Check sheet for the modelled part. Datum: model origin and axes. Units: mm. Face numbers are marked on the shaded views. A direction names the side the tool comes from. Round coordinates to 2 decimals unless told otherwise and drop trailing zeros. Loops run counter-clockwise (first coordinate to the right, second up) from the corner with the lowest first, then second, coordinate; pieces in that order, holes last. Notation, with made-up numbers: (73.5, -18.75) -> (85.5, -18.75) arc R22 ccw to (85.5, -3.75) -> close; hole circle Ø11 at (-39, 24). An arc over 180 degrees is marked (long way). Return JSON: item names as keys, results as strings.
from build123d import *

# Parameters (mm, degrees)
SKETCH2_W           = 61
SKETCH2_H           = 42.5
SKETCH2_R           = 11.5
SKETCH2_R_2         = 1.75
BOSS_EXTRUDE2_DEPTH = 5
BOSS_EXTRUDE3_DEPTH = 3
LPATTERN1_COUNT     = 2
LPATTERN1_PITCH     = 45.5


with BuildPart() as part:
    # Sketch2 → Boss-Extrude2 (new body)
    with BuildSketch(Plane(origin=(0, 0, 0), x_dir=(0, 0, -1), z_dir=(1, 0, 0))):
        with Locations((9.5, 0)):
            Rectangle(SKETCH2_W, SKETCH2_H)
        Circle(SKETCH2_R, mode=Mode.SUBTRACT)
        with Locations((-15.5, 15.5)):
            Circle(SKETCH2_R_2, mode=Mode.SUBTRACT)
        with Locations((15.5, -15.5)):
            Circle(SKETCH2_R_2, mode=Mode.SUBTRACT)
        with Locations((15.5, 15.5)):
            Circle(SKETCH2_R_2, mode=Mode.SUBTRACT)
        with Locations((-15.5, -15.5)):
            Circle(SKETCH2_R_2, mode=Mode.SUBTRACT)
        with BuildLine():
            Line((28.5, 12.75), (31.5, 12.75))
            ThreePointArc((31.5, 12.75), (34.25, 10), (31.5, 7.25))
            Line((31.5, 7.25), (28.5, 7.25))
            ThreePointArc((28.5, 7.25), (25.75, 10), (28.5, 12.75))
        make_face(mode=Mode.SUBTRACT)
        with BuildLine():
            Line((28.5, -12.75), (31.5, -12.75))
            ThreePointArc((31.5, -12.75), (34.25, -10), (31.5, -7.25))
            Line((31.5, -7.25), (28.5, -7.25))
            ThreePointArc((28.5, -7.25), (25.75, -10), (28.5, -12.75))
        make_face(mode=Mode.SUBTRACT)
    extrude(amount=BOSS_EXTRUDE2_DEPTH)

    # Sketch4 → Boss-Extrude3 (add)
    with BuildSketch(Plane.XZ.offset(21.25)):
        Polygon((0, -40), (15, -40), (5, 21), (0, 21), align=None)
    boss_extrude3 = extrude(amount=BOSS_EXTRUDE3_DEPTH)

    # LPattern1: Boss-Extrude3 ×2
    with Locations(*[(0, i * LPATTERN1_PITCH, 0) for i in range(1, LPATTERN1_COUNT)]):
        add(boss_extrude3)


solid = part.part
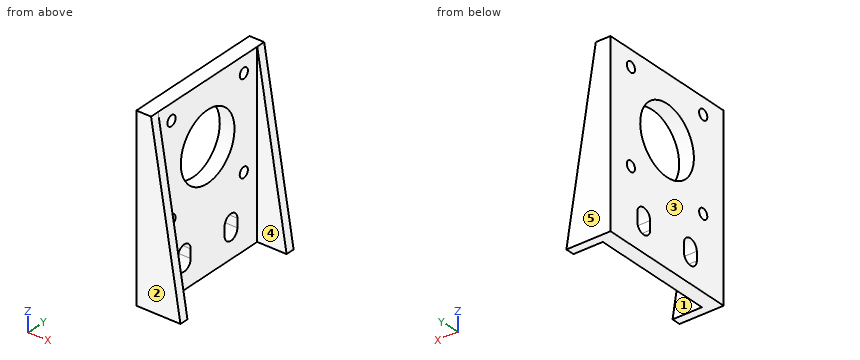
Q1. Section check C-C (x = 4.25). Record the boundary of the cut face in (y, z).
Results list:
{"outline": "(-24.25, -40) -> (24.25, -40) -> (24.25, 21) -> (-24.25, 21) -> close; hole circle Ø3.5 at (-15.5, -15.5); hole circle Ø3.5 at (-15.5, 15.5); hole (-12.75, -31.5) arc R2.75 ccw to (-7.25, -31.5) -> (-7.25, -28.5) arc R2.75 ccw to (-12.75, -28.5) -> close; hole circle Ø23 at (0, 0); hole (7.25, -31.5) arc R2.75 ccw to (12.75, -31.5) -> (12.75, -28.5) arc R2.75 ccw to (7.25, -28.5) -> close; hole circle Ø3.5 at (15.5, -15.5); hole circle Ø3.5 at (15.5, 15.5)"}
Q2. Go/stop test with flat-tipped pins: pin 1 (4.5 mm diameter, centred on y = 15.5, z = -15.5, fed in from +X); pin 2 (4 mm diameter, centred on x = 5.5, y = 6, fed in from +Z). Record where each tip stops, or that it passes through.
Results list:
{"pin 1": "x = 5", "pin 2": "z = 21"}
Q3. Section check B-B (y = 15.5). Record the boundary of the cut face in (x, z).
Results list:
{"outline": "(0, -40) -> (5, -40) -> (5, -17.25) -> (0, -17.25) -> close; (0, -13.75) -> (5, -13.75) -> (5, 13.75) -> (0, 13.75) -> close; (0, 17.25) -> (5, 17.25) -> (5, 21) -> (0, 21) -> close"}
Q4. Material ranges on line 1 (Y direction, x = 3.5, z = -15.5); line 2 (Y direction, x = 2.25, z = -31); line 3 (Y direction, x = 3.25, z = 0), recorded low to high.
Results list:
{"line 1": "-24.25 to -17.25, -13.75 to 13.75, 17.25 to 24.25", "line 2": "-24.25 to -12.75, -7.25 to 7.25, 12.75 to 24.25", "line 3": "-24.25 to -11.5, 11.5 to 24.25"}
Q5. Section check D-D (z = -10.5). Record the boundary of the cut face in (x, y).
Results list:
{"outline": "(0, -24.25) -> (10.16, -24.25) -> (10.16, -21.25) -> (5, -21.25) -> (5, -4.69) -> (0, -4.69) -> close; (0, 4.69) -> (5, 4.69) -> (5, 21.25) -> (10.16, 21.25) -> (10.16, 24.25) -> (0, 24.25) -> close"}
Q6. Section check A-A (x = 8.5). Record the boundary of the cut face in (y, z).
Results list:
{"outline": "(-24.25, -40) -> (-21.25, -40) -> (-21.25, -0.35) -> (-24.25, -0.35) -> close; (21.25, -40) -> (24.25, -40) -> (24.25, -0.35) -> (21.25, -0.35) -> close"}
Q7. Tool access check on the marked faces 1 and 2. Record the directions out of +Z, -Z, +X, -X, +Y, -Y that give a thin tool (end or side, any length) a straight path to the whole face; none if there is none.
Results list:
{"face 1": "+Z, -Z, +X", "face 2": "+Z, -Z, +X, -X, -Y"}
Q8. Draft check along Y on the marked faces 3, 4 and 5. Enter one of: released by +Y, released by -Y, zero draft, split by the parting line, or undercut.
Results list:
{"face 3": "zero draft", "face 4": "undercut", "face 5": "released by +Y"}
